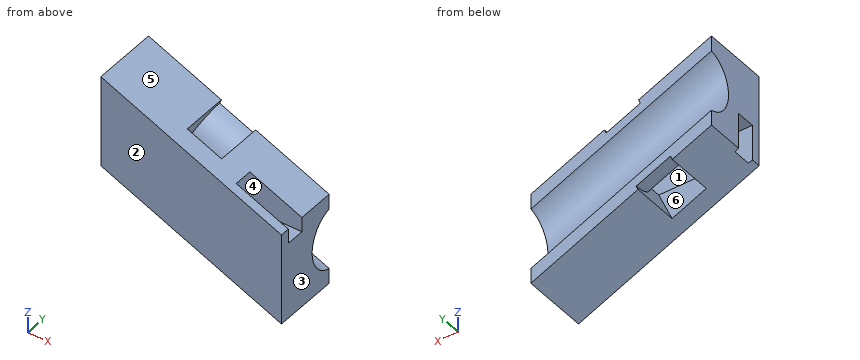
```python
from build123d import *

# Parameters (mm, degrees)
BOSS_EXTRUDE2_DEPTH     = 7
CUT_EXTRUDE4_DEPTH      = 25
CUT_EXTRUDE7_DEPTH      = 4
SKETCH6_W               = 4
SKETCH6_H               = 2
CUT_EXTRUDE5_DEPTH      = 23.912878475
CUT_EXTRUDE5_DEPTH_BACK = 4.6
SKETCH12_W              = 3.6
SKETCH12_H              = 9.819805061
CUT_EXTRUDE10_DEPTH     = 8
SKETCH13_W              = 3.6
SKETCH13_H              = 9.819805061
CUT_EXTRUDE11_DEPTH     = 8


with BuildPart() as part:
    # Sketch2 → Boss-Extrude2 (new body)
    with BuildSketch(Plane(origin=(0, 0, 0), x_dir=(1, 0, 0), z_dir=(0, 1, 0))):
        Polygon((0, 0), (-3.6, 8.248636251), (19.312878475, 18.248636251), (22.912878475, 10), align=None)
    extrude(amount=BOSS_EXTRUDE2_DEPTH)

    # Sketch4 → Cut-Extrude4 (cut)
    with BuildSketch(Plane(origin=(0, 0, 0), x_dir=(0.4, 0, 0.916515139), z_dir=(-0.916515139, 0, 0.4))):
        with BuildLine():
            Line((-7.5, 7), (-1.5, 7))
            ThreePointArc((-1.5, 7), (-4.5, 4.5), (-7.5, 7))
        make_face()
    extrude(amount=-CUT_EXTRUDE4_DEPTH, mode=Mode.SUBTRACT)

    # Sketch8 → Cut-Extrude7 (cut)
    with BuildSketch(Plane(origin=(11.456439237, 0, -5), x_dir=(-0.4, 0, -0.916515139), z_dir=(0.916515139, 0, -0.4))):
        with BuildLine():
            Line((0.48751947, 7), (0, 7))
            Line((0, 7), (0, 2))
            Line((0, 2), (9, 2))
            Line((9, 2), (9, 7))
            Line((9, 7), (8.51248053, 7))
            ThreePointArc((8.51248053, 7), (4.5, 3.5), (0.48751947, 7))
        make_face()
    extrude(amount=-CUT_EXTRUDE7_DEPTH, mode=Mode.SUBTRACT)

    # Sketch6 → Cut-Extrude5 (cut, two sides)
    with BuildSketch(Plane(origin=(0, 0, 0), x_dir=(0, 0, -1), z_dir=(1, 0, 0))) as cut_extrude5_sk:
        with Locations((8, 2)):
            Rectangle(SKETCH6_W, SKETCH6_H)
    extrude(amount=CUT_EXTRUDE5_DEPTH, mode=Mode.SUBTRACT)
    extrude(cut_extrude5_sk.sketch, amount=-CUT_EXTRUDE5_DEPTH_BACK, mode=Mode.SUBTRACT)

    # Sketch12 → Cut-Extrude10 (cut, through all)
    with BuildSketch(Plane(origin=(0, 0, 0), x_dir=(1, 0, 0), z_dir=(0, 1, 0))):
        with Locations((21.112878475, 13.338733721)):
            Rectangle(SKETCH12_W, SKETCH12_H)
    extrude(amount=CUT_EXTRUDE10_DEPTH, mode=Mode.SUBTRACT)

    # Sketch13 → Cut-Extrude11 (cut, through all)
    with BuildSketch(Plane(origin=(0, 0, 0), x_dir=(1, 0, 0), z_dir=(0, 1, 0))):
        with Locations((-1.8, 4.909902531)):
            Rectangle(SKETCH13_W, SKETCH13_H)
    extrude(amount=CUT_EXTRUDE11_DEPTH, mode=Mode.SUBTRACT)


solid = part.part
```
The model under review builds one solid part; all positions refer to its coordinate system, in mm. Face numbers are marked on the shaded views. A direction names the side the tool comes from. Round coordinates to 2 decimals unless told otherwise and drop trailing zeros. Loops run counter-clockwise (first coordinate to the right, second up) from the corner with the lowest first, then second, coordinate; pieces in that order, holes last.
1) Consider section B-B on y = 6. State the section outline as (x, z) points.
Values follow:
outline: (0, -9.82) - (4.19, -11.65) - (4.49, -10.95) - (8.16, -12.55) - (7.86, -13.25) - (19.31, -18.25) - (19.31, -16.2) - (0, -7.78) - close; (0, -2.04) - (19.31, -10.47) - (19.31, -8.43) - (11.46, -5) - (11.15, -5.7) - (7.49, -4.1) - (7.79, -3.4) - (0, 0) - close
2) Consider section D-D on z = -17. State the section outline as (x, y) points.
Values follow:
outline: (16.45, 0) - (19.31, 0) - (19.31, 7) - (16.45, 7) - close
3) Consider section C-C on y = 3.75. State the section outline as (x, z) points, then the cut area to 3 significant figures.
Values follow:
outline: (0, -9.82) - (4.19, -11.65) - (5.43, -8.81) - (9.1, -10.41) - (7.86, -13.25) - (19.31, -18.25) - (19.31, -8.43) - (11.46, -5) - (10.22, -7.84) - (6.55, -6.24) - (7.79, -3.4) - (0, 0) - close
area: 165 mm2
4) Wall thickness on line 1 along Y through (x, z) = (5, -7); line 2 along Z through (x, y) = (3, 2.25); line 3 along Z through (x, y) = (7.25, 6.25): over which ranges is each line inside the solid? List them lowest first.
Values follow:
line 1: y = 0 to 1, 3 to 4.5
line 2: z = -11.13 to -10, -6 to -1.31
line 3: z = -12.26 to -11.08, -5.06 to -3.16
5) Clearance check with flat-ended pins moving along their axes: P1, Ø0.6, axis at x = 8.5, y = 1.5, coming from the -Z side; P2, Ø2, axis at x = 11.5, y = 2, coming from the +Z side; P3, Ø1, axis at x = 5.5, z = -9.5, coming from the +Y side. State where each tip first meets the part, or that it passes through.
Values follow:
P1: stops at z = -13.66
P2: stops at z = -4.58
P3: stops at y = 5.81
6) The part is to be moulded in two halves that separate along Y. For the marked faces 1, 2 and 3, say which applies: pulls with the +Y half, pulls with the -Y half, needs draft (parallel to the pull), parting line crosses it, or undercut.
Values follow:
face 1: undercut
face 2: pulls with the -Y half
face 3: needs draft
7) Tool access review of the marked faces 4, 5 and 6: name each direction out of +Z, -Z, +X, -X, +Y, -Y from which nothing blocks a thin tool from reaching the whole face with its end or side.
Values follow:
face 4: +X, -X
face 5: +Z, +X, +Y, -Y
face 6: none
8) Consider section A-A on y = 1.5. State the section outline as (x, z) points.
Values follow:
outline: (0, -6) - (13.75, -6) - (0, 0) - close; (0.41, -10) - (19.31, -18.25) - (19.31, -10) - close
